from build123d import *

# Parameters (mm, degrees)
SKETCH_R      = 9.2
EXTRUDE_DEPTH = 10


with BuildPart() as part:
    # Sketch → Extrude (new body)
    with BuildSketch(Plane.XY):
        with BuildLine():
            ThreePointArc((-6.022522, 10.839217), (-10.07862, 8.827673), (-8.96, 4.440541))
            ThreePointArc((-8.96, 4.440541), (0, -10), (8.96, 4.440541))
            ThreePointArc((8.96, 4.440541), (10.07862, 8.827673), (6.022522, 10.839217))
            ThreePointArc((6.806908, 7.325709), (7.207742, 9.259505), (6.022522, 10.839217))
            ThreePointArc((6.806908, 7.325709), (0, 10), (-6.806908, 7.325709))
            ThreePointArc((-6.022522, 10.839217), (-7.207742, 9.259505), (-6.806908, 7.325709))
        make_face()
        Circle(SKETCH_R, mode=Mode.SUBTRACT)
    extrude(amount=EXTRUDE_DEPTH)


solid = part.part
Read the model definition and answer for the solid it produces. Units are mm, in the model's axes. A direction names the side the tool comes from. Give positions to 0.01 mm unless a question says otherwise; leave off trailing zeros. Write each loop counter-clockwise with the first axis right and the second up, starting at its lowest first coordinate (ties: lowest second). Pieces come first, ordered by that corner, then holes. Notation, with made-up numbers: (12.5, 4.25) - (47.5, 4.25) arc R28 ccw to (47.5, 24.25) - close; hole circle Ø2 at (39, -7.75). An arc over 180 degrees is marked (long way). Use CSV: the item, a comma, the result in double quotes. Start each with the question number.
Item 1: The part is cut by section A-A, the plane x = 0. Give the vertices of the cut face in (y, z).
Item 2: Flat-ended cylindrical pins translate along their axes: P1, Ø1, axis at y = -6.5, z = 5.5, coming from the -X side; P2, Ø2, axis at x = 6.5, z = 8, coming from the -Y side; P3, Ø2, axis at x = -1, z = 1.5, coming from the +Y side. Find the tip coordinate at first contact, or state that the pin passes through.
Item 3: The part is cut by section C-C, the plane z = 7.25. Give the vertices of the cut face in (x, y).
Item 4: The mould has two halves that part along X. Classify faces 1 (the cylindrical face through (7.214, 9.232, 4.93)), 2 (the flat face through (3, 9, 0)), 3 (the cylindrical face through (0, -10, 5)): pulls with the +X half, pulls with the -X half, needs draft (parallel to the pull), parting line crosses it, or undercut.
Item 5: Consider line 1 (Y direction, x = 0.25, z = 6.5); line 2 (Y direction, x = -6.75, z = 0.75). Determine where each line is inside the solid, lowest interval first.
Item 6: For faces 4 (the cylindrical face through (0, 10, 5)), 5 (the flat face through (3, 9, 10)), determine the directions among +Z, -Z, +X, -X, +Y, -Y from which every point of the face is accessible in a straight line to the end or side of a thin tool.
Taken from the geometry:
1,outline,"(-10, 0) - (-9.2, 0) - (-9.2, 10) - (-10, 10) - close; (9.2, 0) - (10, 0) - (10, 10) - (9.2, 10) - close"
2,P1,"x = -8"
2,P2,"y = -8.35"
2,P3,"y = 10"
3,outline,"(-8.96, 4.44) arc R10 ccw (long way) to (8.96, 4.44) arc R3.6 ccw to (6.02, 10.84) arc R2.4 cw to (6.81, 7.33) arc R10 ccw to (-6.81, 7.33) arc R2.4 cw to (-6.02, 10.84) arc R3.6 ccw to start; hole circle Ø18.4 at (0, 0)"
4,face 1,"undercut"
4,face 2,"needs draft"
4,face 3,"parting line crosses it"
5,line 1,"-10 to -9.2, 9.2 to 10"
5,line 2,"-7.38 to -6.25, 6.25 to 7.38, 10.22 to 10.93"
6,face 4,"+Z, -Z"
6,face 5,"+Z, +X, -X, +Y, -Y"
